Source: three-view drawing plus pictorial views. Frame: mm from the lowest corner of the part. Round coordinates to 2 decimals unless told otherwise and drop trailing zeros. Loops run counter-clockwise (first coordinate to the right, second up) from the corner with the lowest first, then second, coordinate; pieces in that order, holes last. Notation, with made-up numbers: (15, -31.75) -> (25, -31.75) arc R21 cw to (25, 6.25) -> close; hole circle Ø10 at (55.5, -15). An arc over 180 degrees is marked (long way). Answer in a Markdown table with one row per item. Add a question column.
Q1. Mould query, pull axis Z, two halves, no side actions, for the marked faces 1 and 2. Classes: pulls with the +Z half, pulls with the -Z half, needs draft (parallel to the pull), parting line crosses it, or undercut.
Q2. Section B-B, the plane x = 38.1. Output: boundary loops of the cut face in (y, z), and give its area (3 significant figures).
Q3. Section D-D, the plane z = 1.5. Output: boundary loops of the cut face in (x, y), and give its area (3 significant figures).
Q4. Ray query, L1, parallel to Y at x = 38.1, z = 1.75; L2, parallel to X at y = 4, z = 2.35; L3, parallel to Y at x = 48.35, z = 1.3. Return the intervals inside material, ascending. Write a range as from..to.
Q5. Pin query (flat end, axial travel): pin 1 (1.5 mm diameter, centred on y = 22.5, z = 1, fed in from -X); pin 2 (2 mm diameter, centred on x = 38.1, y = 36.304, fed in from +Z); pin 3 (0.8 mm diameter, centred on x = 57, z = 1.5, fed in from +Y). Return the tip coordinate at first contact, or that it passes through.
Q6. Section A-A, the plane x = 27.85. Output: boundary loops of the cut face in (y, z), and give its area (3 significant figures).
Q7. Section C-C, the plane y = 17. Output: boundary loops of the cut face in (x, z), and give its area (3 significant figures).
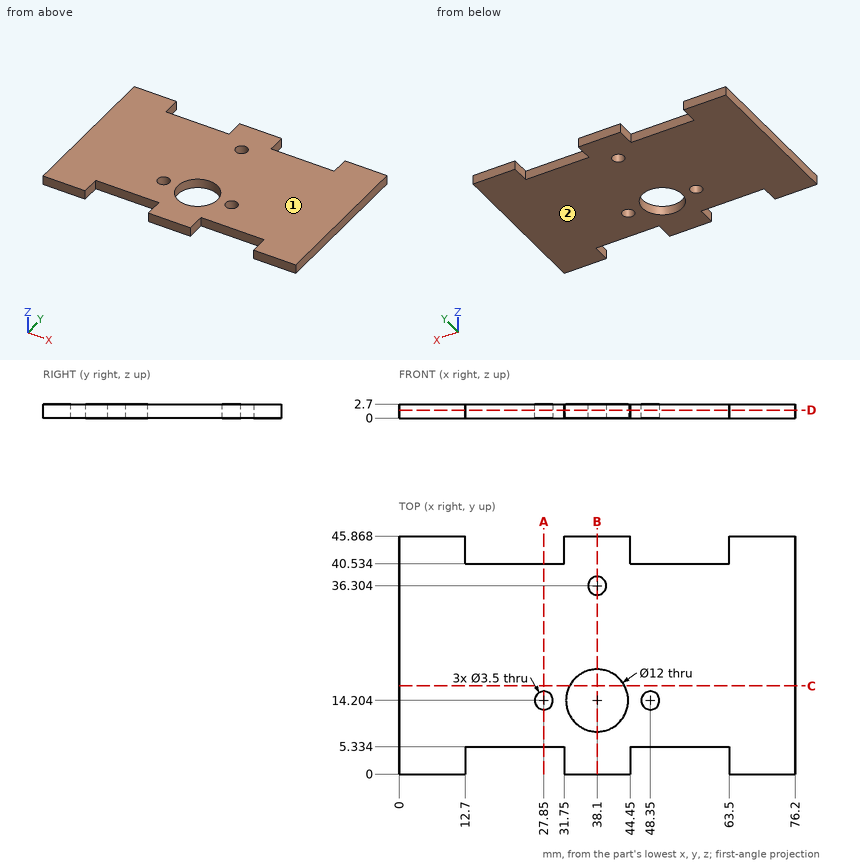
Answer block:
| question | item | result |
|---|---|---|
| 1 | face 1 | pulls with the +Z half |
| 1 | face 2 | pulls with the -Z half |
| 2 | outline | (0, 0) -> (8.2, 0) -> (8.2, 2.7) -> (0, 2.7) -> close; (20.2, 0) -> (34.55, 0) -> (34.55, 2.7) -> (20.2, 2.7) -> close; (38.05, 0) -> (45.87, 0) -> (45.87, 2.7) -> (38.05, 2.7) -> close |
| 2 | area | 82.0 mm^2 |
| 3 | outline | (0, 0) -> (12.7, 0) -> (12.7, 5.33) -> (31.75, 5.33) -> (31.75, 0) -> (44.45, 0) -> (44.45, 5.33) -> (63.5, 5.33) -> (63.5, 0) -> (76.2, 0) -> (76.2, 45.87) -> (63.5, 45.87) -> (63.5, 40.53) -> (44.45, 40.53) -> (44.45, 45.87) -> (31.75, 45.87) -> (31.75, 40.53) -> (12.7, 40.53) -> (12.7, 45.87) -> (0, 45.87) -> close; hole circle Ø3.5 at (27.85, 14.2); hole circle Ø12 at (38.1, 14.2); hole circle Ø3.5 at (38.1, 36.3); hole circle Ø3.5 at (48.35, 14.2) |
| 3 | area | 2,950 mm^2 |
| 4 | L1 | 0..8.2, 20.2..34.55, 38.05..45.87 |
| 4 | L2 | 0..12.7, 31.75..44.45, 63.5..76.2 |
| 4 | L3 | 5.33..12.45, 15.95..40.53 |
| 5 | pin 1 | x = 0 |
| 5 | pin 2 | through |
| 5 | pin 3 | y = 40.53 |
| 6 | outline | (5.33, 0) -> (12.45, 0) -> (12.45, 2.7) -> (5.33, 2.7) -> close; (15.95, 0) -> (40.53, 0) -> (40.53, 2.7) -> (15.95, 2.7) -> close |
| 6 | area | 85.6 mm^2 |
| 7 | outline | (0, 0) -> (32.79, 0) -> (32.79, 2.7) -> (0, 2.7) -> close; (43.41, 0) -> (76.2, 0) -> (76.2, 2.7) -> (43.41, 2.7) -> close |
| 7 | area | 177 mm^2 |
